```python
from build123d import *

# Parameters (mm, degrees)
SZKIC1_W                    = 45
SZKIC1_H                    = 60
SZKIC1_R                    = 4.5
DODANIE_WYCI_GNI_CIE1_DEPTH = 5
SZKIC2_R                    = 6
WYTNIJ_WYCI_GNI_CIE1_DEPTH  = 10


with BuildPart() as part:
    # Szkic1 → Dodanie-wyciągnięcie1 (new body)
    with BuildSketch(Plane.XY):
        Rectangle(SZKIC1_W, SZKIC1_H)
        with Locations((-14.5, 24.5)):
            Circle(SZKIC1_R, mode=Mode.SUBTRACT)
        with Locations((-14.5, -24.5)):
            Circle(SZKIC1_R, mode=Mode.SUBTRACT)
    extrude(amount=DODANIE_WYCI_GNI_CIE1_DEPTH)

    # Szkic2 → Wytnij-wyciągnięcie1 (cut)
    with BuildSketch(Plane.XY.offset(5)):
        with Locations((7.5, 23)):
            Circle(SZKIC2_R)
    extrude(amount=-WYTNIJ_WYCI_GNI_CIE1_DEPTH, mode=Mode.SUBTRACT)


solid = part.part
```
CAD build for the part. Positions are in the model's coordinates, mm. Coordinates: 2 decimals unless noted, no trailing zeros. Order: outer loops, then holes, each group sorted by start corner. A loop starts at its lowest first (then second) coordinate and runs counter-clockwise, first axis right, second up. Notation, with made-up numbers: (30, -33.5) -> (80, -33.5) arc R17 ccw to (80, -25.5) -> close; hole circle Ø5 at (14.25, 42). An arc over 180 degrees is marked (long way). Use one line per item in the form item = value. Start each with the question number.
1) Pull direction Y, two halves, no side cores. Call faces 1 (the cylindrical face through (-17.82, 27.54, 2.46)), 2 (the flat face through (0, 30, 2)), 3 (the flat face through (-22.5, 0, 2)), 4 (the flat face through (0, -30, 2)): +Y half, -Y half, draft (parallel to the pull), parting line (faces both ways), or undercut.
2) Band-saw the part on A-A on x = 7.5. Give the cut face in (y, z), then the cut area to 3 significant figures.
3) Drill centre lines: L1, parallel to Y at x = -14.5, z = 3.95; L2, parallel to Y at x = 7.5, z = 2.9; L3, parallel to Y at x = -10.5, z = 2.35. Where is each one in solid material? Low to high. Write a range as [from, to].
4) Band-saw the part on B-B on z = 4. Give the cut face in (x, y).
5) Band-saw the part on D-D on x = -14.5. Give the cut face in (y, z).
6) Band-saw the part on C-C on y = 24.5. Give the cut face in (x, z), then the cut area to 3 significant figures.
Entries:
q1.face_1 = undercut
q1.face_2 = +Y half
q1.face_3 = draft
q1.face_4 = -Y half
q2.outline = (-30, 0) -> (17, 0) -> (17, 5) -> (-30, 5) -> close; (29, 0) -> (30, 0) -> (30, 5) -> (29, 5) -> close
q2.area = 240 mm2
q3.L1 = [-30, -29], [-20, 20], [29, 30]
q3.L2 = [-30, 17], [29, 30]
q3.L3 = [-30, -26.56], [-22.44, 22.44], [26.56, 30]
q4.outline = (-22.5, -30) -> (22.5, -30) -> (22.5, 30) -> (-22.5, 30) -> close; hole circle Ø9 at (-14.5, -24.5); hole circle Ø9 at (-14.5, 24.5); hole circle Ø12 at (7.5, 23)
q5.outline = (-30, 0) -> (-29, 0) -> (-29, 5) -> (-30, 5) -> close; (-20, 0) -> (20, 0) -> (20, 5) -> (-20, 5) -> close; (29, 0) -> (30, 0) -> (30, 5) -> (29, 5) -> close
q6.outline = (-22.5, 0) -> (-19, 0) -> (-19, 5) -> (-22.5, 5) -> close; (-10, 0) -> (1.69, 0) -> (1.69, 5) -> (-10, 5) -> close; (13.31, 0) -> (22.5, 0) -> (22.5, 5) -> (13.31, 5) -> close
q6.area = 122 mm2
